Check sheet for the modelled part. Datum: model origin and axes. Units: mm. Face numbers are marked on the shaded views. A direction names the side the tool comes from. Coordinates: 2 decimals unless noted, no trailing zeros. Write each loop counter-clockwise with the first axis right and the second up, starting at its lowest first coordinate (ties: lowest second). Pieces come first, ordered by that corner, then holes. Notation, with made-up numbers: M -8,-29 L 25,-29 A20 ccw 25,10 Z; hole C 60.5,-14.5 d10. An arc over 180 degrees is marked long. Answer as CSV lines item,"result".
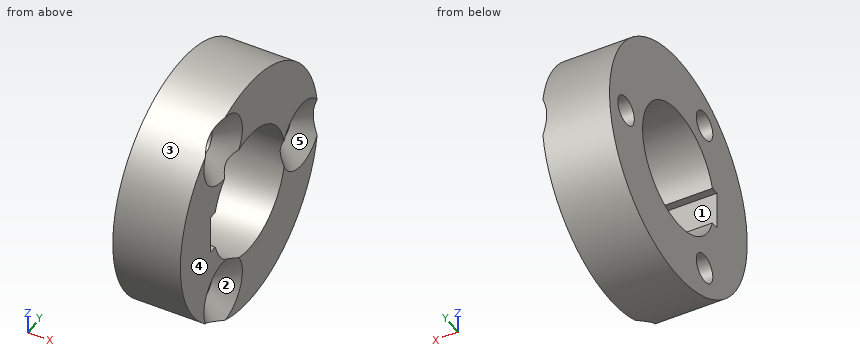
from build123d import *

# Parameters (mm, degrees)
SKETCH1_R           = 12.5
SKETCH1_R_2         = 6.5
SKETCH1_R_3         = 1.5
BOSS_EXTRUDE1_DEPTH = 7
CHAMFER1_SIZE       = 2
SKETCH2_W           = 4
SKETCH2_H           = 4
CUT_EXTRUDE1_DEPTH  = 10


with BuildPart() as part:
    # Sketch1 → Boss-Extrude1 (new body)
    with BuildSketch(Plane(origin=(0, 0, 0), x_dir=(0, 0, -1), z_dir=(1, 0, 0))):
        Circle(SKETCH1_R)
        Circle(SKETCH1_R_2, mode=Mode.SUBTRACT)
        with Locations((0, 9.5)):
            Circle(SKETCH1_R_3, mode=Mode.SUBTRACT)
        with Locations((-8.227241336, -4.75)):
            Circle(SKETCH1_R_3, mode=Mode.SUBTRACT)
        with Locations((8.227241336, -4.75)):
            Circle(SKETCH1_R_3, mode=Mode.SUBTRACT)
    extrude(amount=BOSS_EXTRUDE1_DEPTH)

    # Chamfer1
    # the kernel refuses this chamfer: 2 mm, written as the material it takes off along each edge
    with BuildSketch(Plane(origin=(7, -4.75, 8.227241336), x_dir=(0, 0, -1), z_dir=(0, -1, 0))) as chamfer1_piece_1:
        Polygon((1.5, -CHAMFER1_SIZE), (1.5 + CHAMFER1_SIZE, 0), (1.5, 0), align=None)
    revolve(axis=Axis((7, -4.75, 8.227241336), (1, 0, 0)), mode=Mode.SUBTRACT)
    with BuildSketch(Plane(origin=(7, -4.75, -8.227241336), x_dir=(0, 0, -1), z_dir=(0, -1, 0))) as chamfer1_piece_2:
        Polygon((1.5, -CHAMFER1_SIZE), (1.5 + CHAMFER1_SIZE, 0), (1.5, 0), align=None)
    revolve(axis=Axis((7, -4.75, -8.227241336), (1, 0, 0)), mode=Mode.SUBTRACT)
    with BuildSketch(Plane(origin=(7, 9.5, 0), x_dir=(0, 0, -1), z_dir=(0, -1, 0))) as chamfer1_piece_3:
        Polygon((1.5, -CHAMFER1_SIZE), (1.5 + CHAMFER1_SIZE, 0), (1.5, 0), align=None)
    revolve(axis=Axis((7, 9.5, 0), (1, 0, 0)), mode=Mode.SUBTRACT)

    # Sketch2 → Cut-Extrude1 (cut)
    with BuildSketch(Plane.ZY):
        with Locations((0, -5)):
            Rectangle(SKETCH2_W, SKETCH2_H)
    extrude(amount=-CUT_EXTRUDE1_DEPTH, mode=Mode.SUBTRACT)


solid = part.part
1) Section check A-A, the plane x = 4. Record the boundary of the cut face in (y, z), plus the area to 3 significant figures.
Answer key:
outline,"C 0,0 d25; hole M -7,-2 L -6.18,-2 A6.5 ccw long -6.18,2 L -7,2 Z; hole C -4.75,-8.23 d3; hole C -4.75,8.23 d3; hole C 9.5,0 d3"
area,"335 mm2"
2) Tool access check on the marked faces 1 and 2. Record the directions out of +Z, -Z, +X, -X, +Y, -Y that give a thin tool (end or side, any length) a straight path to the whole face; none if there is none.
Answer key:
face 1,"+X, -X"
face 2,"+X"
3) Section check C-C, the plane y = 0. Record the boundary of the cut face in (x, z).
Answer key:
outline,"M 0,-12.5 L 7,-12.5 L 7,-6.5 L 0,-6.5 Z; M 0,6.5 L 7,6.5 L 7,12.5 L 0,12.5 Z"
4) Section check D-D, the plane y = 9.5. Record the boundary of the cut face in (x, z), plus the area to 3 significant figures.
Answer key:
outline,"M 0,-8.12 L 7,-8.12 L 7,-3.5 L 5,-1.5 L 0,-1.5 Z; M 0,1.5 L 5,1.5 L 7,3.5 L 7,8.12 L 0,8.12 Z"
area,"88.7 mm2"
5) Depth check by flat-ended pin: P1, Ø5, axis at y = -4.75, z = 8.23, coming from the -X side; P2, Ø2, axis at x = 5.5, y = 1.5, coming from the +Z side; P3, Ø5, axis at y = 9.5, z = 0, coming from the +X side; P4, Ø2, axis at x = 1.5, z = 10, coming from the -Y side. Enter the tip coordinate at first touch or a pass-through.
Answer key:
P1,"stops at x = 0"
P2,"stops at z = 12.49"
P3,"stops at x = 6"
P4,"stops at y = -8.67"
6) Section check B-B, the plane z = 0. Record the boundary of the cut face in (x, y).
Answer key:
outline,"M 0,-12.5 L 7,-12.5 L 7,-7 L 0,-7 Z; M 0,6.5 L 6.5,6.5 L 5,8 L 0,8 Z; M 0,11 L 5,11 L 6.5,12.5 L 0,12.5 Z"
7) Thickness scan on line 1 along Y through (x, z) = (2, 0); line 2 along Y through (x, z) = (6, 6); line 3 along Y through (x, z) = (6, 9.25). Record the ranges inside material, lowest first.
Answer key:
line 1,"y = -12.5 to -7, 6.5 to 8, 11 to 12.5"
line 2,"y = -10.97 to -5.89, -3.61 to -2.5, 2.5 to 10.97"
line 3,"y = -8.41 to -7.03, -2.47 to 8.41"
8) Mould release check, pull along Y, two halves, no side actions. Record for the marked faces 3, 4 and 5: pulls with the +Y half, pulls with the -Y half, needs draft (parallel to the pull), parting line crosses it, or undercut.
Answer key:
face 3,"parting line crosses it"
face 4,"needs draft"
face 5,"undercut"
